```python
from build123d import *

# Parameters (mm, degrees)
BOSS_EXTRUDE1_DEPTH = 25.4
SKETCH2_R           = 4
BOSS_EXTRUDE2_DEPTH = 12.7
CHAMFER1_SIZE       = 4.92
CHAMFER2_SIZE       = 4.92
SKETCH3_R           = 1.5875
CUT_EXTRUDE1_DEPTH  = 12.7


with BuildPart() as part:
    # Sketch1 → Boss-Extrude1 (new body)
    with BuildSketch(Plane(origin=(0, 0, 0), x_dir=(0, 0, -1), z_dir=(1, 0, 0))):
        Polygon((12.7, 12.800996681), (-12.7, 12.800996681), (-12.7, 0.100996681), (-27.872338694, 0.100996681), (-27.872338694, 3.275996681), (-15.172338694, 3.275996681), (-15.172338694, 15.4293954), (15.307661306, 15.4293954), (15.307661306, 3.275996681), (28.007661306, 3.275996681), (28.007661306, 0.100996681), (12.7, 0.100996681), align=None)
    extrude(amount=BOSS_EXTRUDE1_DEPTH)

    # Sketch2 → Boss-Extrude2 (add)
    with BuildSketch(Plane.XY.offset(15.172338694)):
        with BuildLine():
            Line((4.687120924, 23.442274476), (4.687120924, 15.4293954))
            Line((4.687120924, 15.4293954), (20.712879076, 15.4293954))
            Line((20.712879076, 15.4293954), (20.712879076, 23.442274476))
            ThreePointArc((20.712879076, 23.442274476), (12.7, 31.455153552), (4.687120924, 23.442274476))
        make_face()
        with Locations((12.7, 23.442274476)):
            Circle(SKETCH2_R, mode=Mode.SUBTRACT)
    extrude(amount=-BOSS_EXTRUDE2_DEPTH)

    # Chamfer1
    # the kernel refuses this chamfer: 4.92 mm, written as the material it adds along each edge
    with BuildSketch(Plane(origin=(4.687120924, 15.4293954, 15.172338694), x_dir=(-0.9996219169112966, -0.027495876610586726, 0), z_dir=(0, 0, -1))) as chamfer1_piece_1_section:
        Polygon((CHAMFER1_SIZE * 0.999621916911, CHAMFER1_SIZE * 0.0274958766106), (-CHAMFER1_SIZE * 0.0274958766106, CHAMFER1_SIZE * 0.999621916911), (0, 0), align=None)
    chamfer1_piece_1 = extrude(amount=12.7, mode=Mode.PRIVATE)
    chamfer1_piece_1 = split(chamfer1_piece_1, bisect_by=Plane(origin=(0, 17.064795435, 8.822338694), z_dir=(1, 0, 0)), keep=Keep.TOP, mode=Mode.PRIVATE)
    add(chamfer1_piece_1)
    with BuildSketch(Plane(origin=(20.712879076, 15.4293954, 15.172338694), x_dir=(0.9996219169112966, -0.02749587661058674, 0), z_dir=(0, 0, -1))) as chamfer1_piece_2_section:
        Polygon((CHAMFER1_SIZE * 0.999621916911, -CHAMFER1_SIZE * 0.0274958766106), (-CHAMFER1_SIZE * 0.0274958766106, -CHAMFER1_SIZE * 0.999621916911), (0, 0), align=None)
    chamfer1_piece_2 = extrude(amount=12.7, mode=Mode.PRIVATE)
    chamfer1_piece_2 = split(chamfer1_piece_2, bisect_by=Plane(origin=(25.4, 17.064795435, 8.822338694), z_dir=(-1, 0, 0)), keep=Keep.TOP, mode=Mode.PRIVATE)
    add(chamfer1_piece_2)

    # Chamfer2
    # the kernel refuses this chamfer: 4.92 mm, written as the material it adds along each edge
    with BuildSketch(Plane(origin=(25.4, 15.4293954, 2.472338694), x_dir=(0, -0.02749587661026744, -0.9996219169113054), z_dir=(-1, 0, 0))) as chamfer2_piece_1_section:
        Polygon((CHAMFER2_SIZE * 0.999621916911, -CHAMFER2_SIZE * 0.0274958766106), (-CHAMFER2_SIZE * 0.0274958766103, -CHAMFER2_SIZE * 0.999621916911), (0, 0), align=None)
    chamfer2_piece_1 = extrude(amount=25.4, mode=Mode.PRIVATE)
    chamfer2_piece_1 = split(chamfer2_piece_1, bisect_by=Plane(origin=(23.520525821, 17.541748655, 0.607229555), z_dir=(-0.7071067811868302, -0.7071067811862649, 0)), keep=Keep.TOP, mode=Mode.PRIVATE)
    chamfer2_piece_1 = split(chamfer2_piece_1, bisect_by=Plane(origin=(20.712879076, 16.594460185, 0.607229555), z_dir=(1, 0, 0)), keep=Keep.TOP, mode=Mode.PRIVATE)
    add(chamfer2_piece_1)
    with BuildSketch(Plane(origin=(25.4, 15.4293954, 2.472338694), x_dir=(0, -0.02749587661026744, -0.9996219169113054), z_dir=(-1, 0, 0))) as chamfer2_piece_2_section:
        Polygon((CHAMFER2_SIZE * 0.999621916911, -CHAMFER2_SIZE * 0.0274958766106), (-CHAMFER2_SIZE * 0.0274958766103, -CHAMFER2_SIZE * 0.999621916911), (0, 0), align=None)
    chamfer2_piece_2 = extrude(amount=25.4, mode=Mode.PRIVATE)
    chamfer2_piece_2 = split(chamfer2_piece_2, bisect_by=Plane(origin=(7.03196097, 22.694235446, 0.836220955), z_dir=(0.7071067811868302, -0.7071067811862649, 0)), keep=Keep.TOP, mode=Mode.PRIVATE)
    chamfer2_piece_2 = split(chamfer2_piece_2, bisect_by=Plane(origin=(4.687120924, 17.026196416, 0.836220955), z_dir=(1, 0, 0)), keep=Keep.TOP, mode=Mode.PRIVATE)
    chamfer2_piece_2 = split(chamfer2_piece_2, bisect_by=Plane(origin=(20.712879076, 17.026196416, 0.836220955), z_dir=(-1, 0, 0)), keep=Keep.TOP, mode=Mode.PRIVATE)
    chamfer2_piece_2 = chamfer2_piece_2 - Plane(origin=(12.7, 23.442274476, 0.836220955), x_dir=(1, 0, 0), z_dir=(0, 0, 1)) * Cylinder(4, 71, mode=Mode.PRIVATE)
    add(chamfer2_piece_2)
    with BuildSketch(Plane(origin=(25.4, 15.4293954, 2.472338694), x_dir=(0, -0.02749587661026744, -0.9996219169113054), z_dir=(-1, 0, 0))) as chamfer2_piece_3_section:
        Polygon((CHAMFER2_SIZE * 0.999621916911, -CHAMFER2_SIZE * 0.0274958766106), (-CHAMFER2_SIZE * 0.0274958766103, -CHAMFER2_SIZE * 0.999621916911), (0, 0), align=None)
    chamfer2_piece_3 = extrude(amount=25.4, mode=Mode.PRIVATE)
    chamfer2_piece_3 = split(chamfer2_piece_3, bisect_by=Plane(origin=(1.879474179, 17.541748655, 0.607229555), z_dir=(0.7071067811868302, -0.7071067811862649, 0)), keep=Keep.TOP, mode=Mode.PRIVATE)
    chamfer2_piece_3 = split(chamfer2_piece_3, bisect_by=Plane(origin=(4.687120924, 16.594460185, 0.607229555), z_dir=(-1, 0, 0)), keep=Keep.TOP, mode=Mode.PRIVATE)
    add(chamfer2_piece_3)

    # Sketch3 → Cut-Extrude1 (cut)
    with BuildSketch(Plane(origin=(0, 3.275996681, 0), x_dir=(1, 0, 0), z_dir=(0, 1, 0))):
        with Locations(Location((12.7, 21.657661306, 0), (0, 0, 270))):
            Circle(SKETCH3_R)
        with Locations(Location((12.7, -21.522338694, 0), (0, 0, 270))):
            Circle(SKETCH3_R)
    extrude(amount=-CUT_EXTRUDE1_DEPTH, mode=Mode.SUBTRACT)


solid = part.part
```
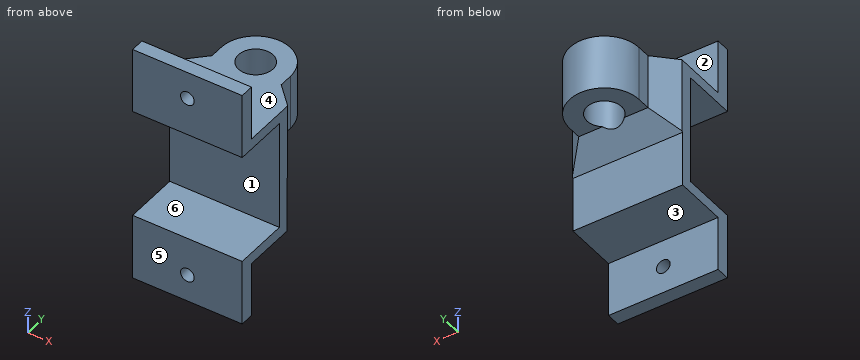
Geometry: final body of the model. Coordinates: model frame, mm. Face numbers are marked on the shaded views. A direction names the side the tool comes from. Round coordinates to 2 decimals unless told otherwise and drop trailing zeros. Write each loop counter-clockwise with the first axis right and the second up, starting at its lowest first coordinate (ties: lowest second). Pieces come first, ordered by that corner, then holes. Notation, with made-up numbers: (15.25, 87.5) -> (48.25, 87.5) arc R16 cw to (48.25, 109.5) -> close; hole circle Ø4 at (-10, 66). An arc over 180 degrees is marked (long way). Return JSON: item names as keys, results as strings.
Q1. Section B-B on y = 25.5. Return the cut outline in (x, z).
From the geometry:
{"outline": "(4.96, 2.47) -> (9.27, 2.47) -> (9.27, 15.17) -> (4.96, 15.17) -> close; (16.13, 2.47) -> (20.44, 2.47) -> (20.44, 15.17) -> (16.13, 15.17) -> close"}
Q2. Ray query, line 1 (Z direction, x = 11.75, y = 8); line 2 (Z direction, x = 2.75, y = 3); line 3 (Y direction, x = 12.7, z = 8.25). Return the intervals inside material, ascending.
From the geometry:
{"line 1": "-15.31 to -12.7, 12.7 to 15.17", "line 2": "-28.01 to -12.7, 12.7 to 27.87", "line 3": "12.8 to 19.44, 27.44 to 31.46"}
Q3. Section C-C on z = -22. Return the cut outline in (x, y), and give its area (3 significant figures).
From the geometry:
{"outline": "(0, 0.1) -> (11.15, 0.1) -> (11.15, 3.28) -> (0, 3.28) -> close; (14.25, 0.1) -> (25.4, 0.1) -> (25.4, 3.28) -> (14.25, 3.28) -> close", "area": "70.8 mm2"}
Q4. Mould query, pull axis Z, two halves, no side actions, for the marked faces 4, 5 and 6. Classes: +Z half, -Z half, draft (parallel to the pull), parting line (faces both ways), or undercut.
From the geometry:
{"face 4": "+Z half", "face 5": "draft", "face 6": "undercut"}
Q5. Set-up query: the marked faces 1, 2 and 3. Return all of +Z, -Z, +X, -X, +Y, -Y with unobstructed straight access to the full face (end or side cutting, diameter ignored); none if empty.
From the geometry:
{"face 1": "+X, -X, -Y", "face 2": "+Z, +X, -X, +Y", "face 3": "-Z, +X, -X, +Y"}
Q6. Section A-A on x = 12.7. Return the cut outline in (y, z), and give its area (3 significant figures).
From the geometry:
{"outline": "(0.1, -28.01) -> (3.28, -28.01) -> (3.28, -23.25) -> (0.1, -23.25) -> close; (0.1, -20.07) -> (3.28, -20.07) -> (3.28, -15.31) -> (15.43, -15.31) -> (15.43, -2.45) -> (19.44, 1.57) -> (19.44, 15.17) -> (3.28, 15.17) -> (3.28, 19.93) -> (0.1, 19.93) -> (0.1, 12.7) -> (12.8, 12.7) -> (12.8, -12.7) -> (0.1, -12.7) -> close; (0.1, 23.11) -> (3.28, 23.11) -> (3.28, 27.87) -> (0.1, 27.87) -> close; (27.44, 2.47) -> (31.46, 2.47) -> (31.46, 15.17) -> (27.44, 15.17) -> close", "area": "319 mm2"}
Q7. First-contact query: pin 1 Ø1 at (x, z) = (15, 19.5) entering from +Y; pin 2 Ø9.5 at (x, y) = (8.5, 11) entering from -Z; pin 3 Ø12 at (x, z) = (9, 1) entering from -Y; pin 4 Ø1 at (y, z) = (13.5, -5) entering from -X. Flat tips, straight axial feed; report the tip coordinate or a pass-through.
From the geometry:
{"pin 1": "y = 3.28", "pin 2": "z = -15.31", "pin 3": "y = 12.8", "pin 4": "x = 0"}
Q8. Section D-D on z = 9. Return the cut outline in (x, y), and give its area (3 significant figures).
From the geometry:
{"outline": "(0, 12.8) -> (25.4, 12.8) -> (25.4, 15.66) -> (20.71, 20.35) -> (20.71, 23.44) arc R8.01 ccw to (4.69, 23.44) -> (4.69, 20.35) -> (0, 15.66) -> close; hole circle Ø8 at (12.7, 23.44)", "area": "270 mm2"}
